Autodesk Inventor part; units mm, degrees
ref_plane "YZ Plane" through (0, 0, 0) normal (1, 0, 0) x (0, 1, 0)
ref_plane "XZ Plane" through (0, 0, 0) normal (0, 1, 0) x (-1, 0, 0)
ref_plane "XY Plane" through (0, 0, 0) normal (0, 0, 1) x (1, 0, 0)
sketch "Sketch1" plane through (0, 0, 0) normal (0, 1, 0) x (-1, 0, 0)
  line L0 (-140, 10) -> (-10, 10)
  line L1 (-10, 10) -> (-10, -10)
  line L2 (-10, -10) -> (-140, -10)
  line L3 (-140, -10) -> (-140, 10)
  line L4 (-140, 10) -> (-10, -10) construction
  line L5 (-10, 10) -> (-140, -10) construction
  line L6 (10, 40) -> (-10, 40)
  line L7 (-10, 40) -> (-10, -40)
  line L8 (-10, -40) -> (10, -40)
  line L9 (10, -40) -> (10, 40)
  line L10 (10, 40) -> (-10, -40) construction
  line L11 (-10, 40) -> (10, -40) construction
  line L12 (40, 0) -> (-170, 0)
  line L13 (0, -56) -> (0, 56)
  circle A0 centre (-15, 0) radius 25
  circle A1 centre (0, 34) radius 4
  circle A2 centre (0, -34) radius 4
  point P0 (0, 0)
  point P1 (-75, 0)
  point P2 (0, 0)
  point P3 (-75, 0)
  point P4 (0, 0)
  point P5 (0, 0)
  point P6 (-37.9129, -10)
  point P7 (-10, -24.4949)
  point P8 (-10, 24.4949)
  point P9 (-37.9129, 10)
  dimension "d0" = 20
  dimension "d1" = 20
  dimension "d2" = 80
  dimension "d3" = 150
  dimension "d5" = 50
  dimension "d6" = 15
  dimension "d7" = 8
  dimension "d8" = 6
  dimension "d9" = 8
  dimension "d10" = 6
extrude "Extrusion1" add sketch "Sketch1" along normal blind 5 contours L0 A0 L12 L3 | A0 L7 L0 | L0 L1 L12 A0 | L12 A0 L2 L3 | L7 A0 L13 L12 L1 | L7 L6 L13 A1 A0 | L12 L1 L2 A0 | L12 L13 A0 L7 L1 | A0 L12 L13 | L13 A1 L6 L9 A0 | L2 L7 A0 | L12 A0 L13 | L9 L8 L13 A2 A0 | A0 L13 A2 L8 L7
equation "\"d0\" = AnEsl"
equation "\"d1\" = AnEsl"
equation "\"d9\" = d7"
equation "\"d10\" = d8"
equation "\"AnEsl\" = 20"
properties part number "T"
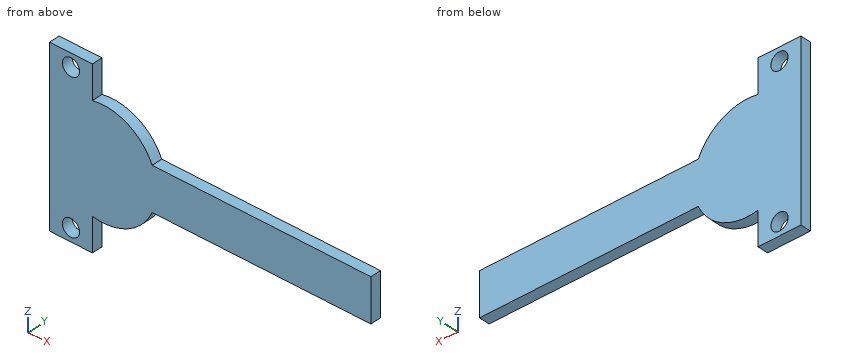
Design review of the part built by this model. Coordinates are the model's own, in mm. Round coordinates to 2 decimals unless told otherwise and drop trailing zeros. Loops run counter-clockwise (first coordinate to the right, second up) from the corner with the lowest first, then second, coordinate; pieces in that order, holes last. Notation, with made-up numbers: (-21.5, 76) - (-16.5, 76) arc R18 cw to (-16.5, 111) - close; hole circle Ø9 at (12.5, 10). An arc over 180 degrees is marked (long way). One line per item, written item: value. Start each with the question number.
1) Consider section B-B on y = 1.9. Give the boundary of the cut face in (x, z).
2) To check wall thickness, follow L1, parallel to Z at x = 0, y = 2.25; L2, parallel to X at y = 1.85, z = -34; L3, parallel to Z at x = 116.5, y = 0.7. State the ranges of each line that lie inside material, in increasing order. Write a range as from..to.
3) Consider section D-D on x = 22. Give the boundary of the cut face in (y, z).
4) Insertion check: pin 1 Ø3 at (y, z) = (3, -24) entering from +X; pin 2 Ø3 at (y, z) = (1, 13.5) entering from +X; pin 3 Ø1.5 at (x, y) = (86, 3) entering from -Z. Each pin has a flat end and moves straight along its axis. Give the tip position at first contact, or say it passes through.
5) Consider section A-A on z = -34. Give the boundary of the cut face in (x, y), then the cut area to 3 significant figures.
6) Consider section C-C on x = 0. Give the boundary of the cut face in (y, z).
Reported:
1. outline: (-10, -40) - (10, -40) - (10, -24.49) arc R25 ccw to (37.91, -10) - (140, -10) - (140, 10) - (37.91, 10) arc R25 ccw to (10, 24.49) - (10, 40) - (-10, 40) - close; hole circle Ø8 at (0, -34); hole circle Ø8 at (0, 34)
2. L1: z = -40..-38, -30..30, 38..40
2. L2: x = -10..-4, 4..10
2. L3: z = -10..10
3. outline: (0, -24) - (5, -24) - (5, 24) - (0, 24) - close
4. pin 1: stops at x = 25.9
4. pin 2: stops at x = 36.93
4. pin 3: stops at z = -10
5. outline: (-10, 0) - (-4, 0) - (-4, 5) - (-10, 5) - close; (4, 0) - (10, 0) - (10, 5) - (4, 5) - close
5. area: 60.0 mm^2
6. outline: (0, -40) - (5, -40) - (5, -38) - (0, -38) - close; (0, -30) - (5, -30) - (5, 30) - (0, 30) - close; (0, 38) - (5, 38) - (5, 40) - (0, 40) - close
